Here's the drawing with two shaded views (mm, measured from the low corner). I have some questions. A direction names the side the tool comes from. Coordinates: 2 decimals unless noted, no trailing zeros. Loops run counter-clockwise (first coordinate to the right, second up) from the corner with the lowest first, then second, coordinate; pieces in that order, holes last. Notation, with made-up numbers: (-14.5, -40) - (14.5, -40) arc R19 ccw to (14.5, -29) - close; hole circle Ø10 at (31.5, 69). An arc over 180 degrees is marked (long way). Use a Markdown table: item, result.
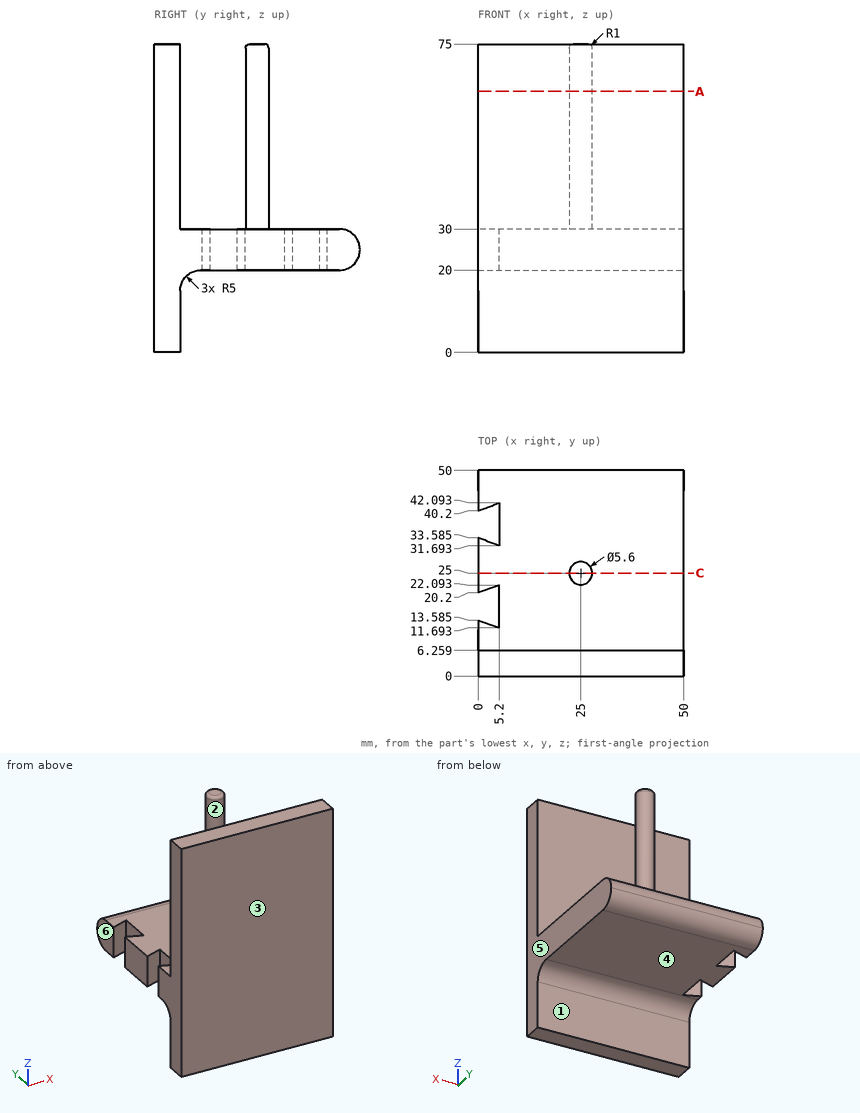
Q1. Will these pins go through, and if not, where does the flat tip stop? P1, Ø12, axis at x = 34, y = 33.5, coming from the -Z side; P2, Ø2, axis at y = 40.5, z = 18, coming from the +X side; P3, Ø22.5, axis at x = 17, z = 61.5, coming from the +Y side; P4, Ø5, axis at x = 29.5, y = 21, coming from the +Z side.
Check values:
| item | result |
|---|---|
| P1 | z = 20 |
| P2 | through |
| P3 | y = 27.8 |
| P4 | z = 30 |
Q2. Please list where these lines run through material, in increasing order: L1, parallel to Y at x = 22, z = 39; L2, parallel to Z at x = 42.5, y = 26; L3, parallel to Y at x = 14.5, z = 25.5 (1 decimal). Write a range as from..to.
Check values:
| item | result |
|---|---|
| L1 | 0..6.26 |
| L2 | 20..30 |
| L3 | 0..50 |
Q3. Which directions (+Z, -Z, +X, -X, +Y, -Y) give clear straight access to the entire face, cutting with the end or side of a thin tool? Please do the marked faces 1, 2 and 3.
Check values:
| item | result |
|---|---|
| face 1 | -Z, +X, -X, +Y |
| face 2 | +Z |
| face 3 | +Z, -Z, +X, -X, -Y |
Q4. I want a section at A-A, the plane z = 63.5. Write out the boundary of the cut face in (x, y).
Check values:
| item | result |
|---|---|
| outline | (0, 0) - (50, 0) - (50, 6.26) - (0, 6.26) - close; circle Ø5.6 at (25, 25) |
Q5. I want a section at C-C, the plane y = 25. Write out the boundary of the cut face in (x, z).
Check values:
| item | result |
|---|---|
| outline | (0, 20) - (50, 20) - (50, 30) - (27.8, 30) - (27.8, 74) arc R1 ccw to (26.8, 75) - (23.2, 75) arc R1 ccw to (22.2, 74) - (22.2, 30) - (0, 30) - close |
Q6. If we mould it in two halves opening along X, with no side actions, what happens to the marked faces 4, 5 and 6? For each: pulls with the +X half, pulls with the -X half, needs draft (parallel to the pull), parting line crosses it, or undercut.
Check values:
| item | result |
|---|---|
| face 4 | needs draft |
| face 5 | pulls with the +X half |
| face 6 | pulls with the -X half |
